from build123d import *

# Parameters (mm, degrees)
SKETCH1_R           = 20
SKETCH1_R_2         = 6
BOSS_EXTRUDE1_DEPTH = 2.5
BOSS_EXTRUDE2_DEPTH = 7.5


with BuildPart() as part:
    # Sketch1 → Boss-Extrude1 (new, symmetric)
    # profile 1 of 2: a face of its own
    with BuildSketch(Plane.XY):
        with BuildLine():
            Line((268.913125513, 20), (0, 20))
            ThreePointArc((0, 20), (14.142135624, 14.142135624), (20, 0))
            ThreePointArc((20, 0), (14.142135624, -14.142135624), (0, -20))
            Line((0, -20), (268.913125513, -20))
            ThreePointArc((268.913125513, -20), (279.827228639, -22.055727726), (289.245570139, -27.941176471))
            ThreePointArc((289.245570139, -27.941176471), (277, 0), (289.245570139, 27.941176471))
            ThreePointArc((289.245570139, 27.941176471), (279.827228639, 22.055727726), (268.913125513, 20))
        make_face()
    # profile 2 of 2: a face of its own
    with BuildSketch(Plane.XY):
        Circle(SKETCH1_R)
        Circle(SKETCH1_R_2, mode=Mode.SUBTRACT)
    extrude(amount=BOSS_EXTRUDE1_DEPTH, both=True)

    # Sketch1_4 → Boss-Extrude2 (add, symmetric)
    with BuildSketch(Plane.XY):
        with BuildLine():
            ThreePointArc((348.730549951, 17.5), (321.56956349, 37.427808319), (289.245570139, 27.941176471))
            ThreePointArc((289.245570139, 27.941176471), (277, 0), (289.245570139, -27.941176471))
            ThreePointArc((289.245570139, -27.941176471), (321.56956349, -37.427808319), (348.730549951, -17.5))
            Line((348.730549951, -17.5), (318.146428929, -17.5))
            ThreePointArc((318.146428929, -17.5), (312.855462018, -9.451474044), (311, 0))
            ThreePointArc((311, 0), (312.855462018, 9.451474044), (318.146428929, 17.5))
            Line((318.146428929, 17.5), (348.730549951, 17.5))
        make_face()
    extrude(amount=BOSS_EXTRUDE2_DEPTH, both=True)


solid = part.part
Could you check a few things on this model? Use its own coordinates, in mm. A direction names the side the tool comes from. Give positions to 0.01 mm unless a question says otherwise; leave off trailing zeros. Order: outer loops, then holes, each group sorted by start corner. A loop starts at its lowest first (then second) coordinate and runs counter-clockwise, first axis right, second up. Notation, with made-up numbers: (15.5, 42.5) -> (56.5, 42.5) arc R14 cw to (56.5, 46.5) -> close; hole circle Ø5 at (0.25, -7.75). An arc over 180 degrees is marked (long way). Answer in a Markdown table with one row per item. Add a question column.
Item 1: Imagine slicing it at D-D (x = 121.5). List the corners of the cut face in (y, z) for me, and give its area (3 significant figures).
Item 2: We'd pull the mould along Y, two halves only. Please class faces 3 (the cylindrical face through (311, 0, 0)), 4 (the cylindrical face through (-20, 0, 0)), 5 (the flat face through (304, 1, 7.5)), 6 (the cylindrical face through (279.68, -22, 0.04)): pulls with the +Y half, pulls with the -Y half, needs draft (parallel to the pull), parting line crosses it, or undercut.
Item 3: I'm going to push flat-ended pins straight in: P1, Ø1, axis at x = 294, z = -2.5, coming from the +Y side; P2, Ø17, axis at x = 135.5, y = 11.5, coming from the -Z side; P3, Ø5.5, axis at x = 139, z = -1, coming from the +Y side; P4, Ø7, axis at x = 0, y = 0, coming from the -Z side. Where does each tip first touch, or does it pass through?
Item 4: Please list where these lines run through material, in increasing order: probe 1 along Y at (x, z) = (0, -0.95); probe 2 along Y at (x, z) = (251.5, 2); probe 3 along Z at (x, y) = (60, -17).
Item 5: Imagine slicing it at B-B (z = 0.25). List the corners of the cut face in (x, y) for me.
Item 6: For faces 1 (the cylindrical face through (279.97, 22.11, 0.04)), 2 (the flat face through (334, -17.5, 0)), which set-ups out of +Z, -Z, +X, -X, +Y, -Y let a thin tool reach every point of the face, with its end or its side?
Item 7: Imagine slicing it at A-A (y = 0). List the corners of the cut face in (x, z) for me, and give its area (4 significant figures).
Item 8: Imagine slicing it at C-C (x = 315). List the corners of the cut face in (y, z) for me.
Result:
| question | item | result |
|---|---|---|
| 1 | outline | (-20, -2.5) -> (20, -2.5) -> (20, 2.5) -> (-20, 2.5) -> close |
| 1 | area | 200 mm2 |
| 2 | face 3 | undercut |
| 2 | face 4 | parting line crosses it |
| 2 | face 5 | needs draft |
| 2 | face 6 | pulls with the -Y half |
| 3 | P1 | y = 32 |
| 3 | P2 | z = -2.5 |
| 3 | P3 | y = 20 |
| 3 | P4 | through |
| 4 | probe 1 | -20 to -6, 6 to 20 |
| 4 | probe 2 | -20 to 20 |
| 4 | probe 3 | -2.5 to 2.5 |
| 5 | outline | (0, -20) -> (268.91, -20) arc R30 cw to (289.25, -27.94) arc R38 ccw to (348.73, -17.5) -> (318.15, -17.5) arc R25 cw to (318.15, 17.5) -> (348.73, 17.5) arc R38 ccw to (289.25, 27.94) arc R30 cw to (268.91, 20) -> (0, 20) arc R20 ccw to start; hole circle Ø12 at (0, 0) |
| 6 | face 1 | +Z, -Z, -X, +Y |
| 6 | face 2 | +Z, -Z, +X |
| 7 | outline | (-20, -2.5) -> (-6, -2.5) -> (-6, 2.5) -> (-20, 2.5) -> close; (6, -2.5) -> (277, -2.5) -> (277, -7.5) -> (311, -7.5) -> (311, 7.5) -> (277, 7.5) -> (277, 2.5) -> (6, 2.5) -> close |
| 7 | area | 1,935 mm2 |
| 8 | outline | (-38, -7.5) -> (-13.56, -7.5) -> (-13.56, 7.5) -> (-38, 7.5) -> close; (13.56, -7.5) -> (38, -7.5) -> (38, 7.5) -> (13.56, 7.5) -> close |
